Read the model definition and answer for the solid it produces. Units are mm, in the model's axes. A direction names the side the tool comes from. Round coordinates to 2 decimals unless told otherwise and drop trailing zeros. Write each loop counter-clockwise with the first axis right and the second up, starting at its lowest first coordinate (ties: lowest second). Pieces come first, ordered by that corner, then holes. Notation, with made-up numbers: (55.5, 18.25) -> (69.5, 18.25) arc R35 cw to (69.5, 54.25) -> close; hole circle Ø11 at (88.25, -37). An arc over 180 degrees is marked (long way). Return JSON: item names as keys, results as strings.
from build123d import *

# Parameters (mm, degrees)
SKETCH1_W             = 76
SKETCH1_H             = 62
BOSS_EXTRUDE1_DEPTH   = 2
SKETCH2_W             = 82
SKETCH2_H             = 68
BOSS_EXTRUDE2_DEPTH   = 8
SKETCH3_W             = 45
SKETCH3_H             = 12.8
CUT_EXTRUDE1_DEPTH    = 11
SKETCH4_R             = 1.6
CUT_EXTRUDE2_DEPTH    = 11
SKETCH5_R             = 3.1
CUT_EXTRUDE3_DEPTH    = 3
SKETCH9_OUTSIDE_W     = 105.4
SKETCH9_OUTSIDE_H     = 91.4
SKETCH9_OUTSIDE_W_2   = 75.6
SKETCH9_OUTSIDE_H_2   = 61.6
CUT_EXTRUDE5_DEPTH    = 3
CUT_EXTRUDE6_DEPTH    = 3
SKETCH11_W            = 66
SKETCH11_H            = 54
CUT_EXTRUDE7_DEPTH    = 7
CHAMFER2_SIZE         = 2
CHAMFER2_SIZE2        = 0.352653961
CHAMFER2_PART_2_SIZE  = 2
CHAMFER2_PART_2_SIZE2 = 0.352653961
CHAMFER3_SIZE         = 1
CHAMFER3_SIZE2        = 1.732050808


with BuildPart() as part:
    # Sketch1 → Boss-Extrude1 (new body)
    with BuildSketch(Plane(origin=(0, 0, 0), x_dir=(1, 0, 0), z_dir=(0, 1, 0))):
        Rectangle(SKETCH1_W, SKETCH1_H)
    extrude(amount=BOSS_EXTRUDE1_DEPTH)

    # Sketch2 → Boss-Extrude2 (add)
    with BuildSketch(Plane(origin=(0, 2, 0), x_dir=(1, 0, 0), z_dir=(0, 1, 0))):
        Rectangle(SKETCH2_W, SKETCH2_H)
    extrude(amount=BOSS_EXTRUDE2_DEPTH)

    # Sketch3 → Cut-Extrude1 (cut, through all)
    with BuildSketch(Plane.XZ):
        with Locations((0, -12.5)):
            Rectangle(SKETCH3_W, SKETCH3_H)
        with Locations((0, 12.5)):
            Rectangle(SKETCH3_W, SKETCH3_H)
    extrude(amount=-CUT_EXTRUDE1_DEPTH, mode=Mode.SUBTRACT)

    # Sketch4 → Cut-Extrude2 (cut, through all)
    with BuildSketch(Plane(origin=(0, 10, 0), x_dir=(1, 0, 0), z_dir=(0, 1, 0))):
        with Locations(Location((-35.408866178, 29.363450001, 0), (0, 0, 270))):  # turned: the seam where the file's is
            Circle(SKETCH4_R)
        with Locations(Location((35.408866178, 29.363450001, 0), (0, 0, 270))):  # turned: the seam where the file's is
            Circle(SKETCH4_R)
        with Locations(Location((35.408866178, -29.363450001, 0), (0, 0, 270))):  # turned: the seam where the file's is
            Circle(SKETCH4_R)
        with Locations(Location((-35.408866178, -29.363450001, 0), (0, 0, 270))):  # turned: the seam where the file's is
            Circle(SKETCH4_R)
    extrude(amount=-CUT_EXTRUDE2_DEPTH, mode=Mode.SUBTRACT)

    # Sketch5 → Cut-Extrude3 (cut)
    with BuildSketch(Plane(origin=(0, 10, 0), x_dir=(1, 0, 0), z_dir=(0, 1, 0))):
        with Locations(Location((-35.408866178, 29.363450001, 0), (0, 0, 270))):  # turned: the seam where the file's is
            Circle(SKETCH5_R)
        with Locations(Location((35.408866178, 29.363450001, 0), (0, 0, 270))):  # turned: the seam where the file's is
            Circle(SKETCH5_R)
        with Locations(Location((35.408866178, -29.363450001, 0), (0, 0, 270))):  # turned: the seam where the file's is
            Circle(SKETCH5_R)
        with Locations(Location((-35.408866178, -29.363450001, 0), (0, 0, 270))):  # turned: the seam where the file's is
            Circle(SKETCH5_R)
    extrude(amount=-CUT_EXTRUDE3_DEPTH, mode=Mode.SUBTRACT)

    # Sketch9 outside → Cut-Extrude5 (cut)
    with BuildSketch(Plane.XZ):
        Rectangle(SKETCH9_OUTSIDE_W, SKETCH9_OUTSIDE_H)
        Rectangle(SKETCH9_OUTSIDE_W_2, SKETCH9_OUTSIDE_H_2, mode=Mode.SUBTRACT)
    extrude(amount=-CUT_EXTRUDE5_DEPTH, mode=Mode.SUBTRACT)

    # Sketch10 → Cut-Extrude6 (cut)
    with BuildSketch(Plane.XZ):
        Polygon((-37.8, -30.8), (-31.8, -30.8), (-37.8, -24.8), align=None)
        Polygon((-37.8, 24.8), (-37.8, 30.8), (-31.8, 30.8), align=None)
        Polygon((37.8, 30.8), (37.8, 24.8), (31.8, 30.8), align=None)
        Polygon((37.8, -30.8), (31.8, -30.8), (37.8, -24.8), align=None)
    extrude(amount=-CUT_EXTRUDE6_DEPTH, mode=Mode.SUBTRACT)

    # Sketch11 → Cut-Extrude7 (cut)
    with BuildSketch(Plane.XZ):
        Rectangle(SKETCH11_W, SKETCH11_H)
    extrude(amount=-CUT_EXTRUDE7_DEPTH, mode=Mode.SUBTRACT)

    # Chamfer2
    chamfer2_edges = [part.edges().sort_by_distance(p)[0] for p in [
        (37.8, 0, 0),
    ]]
    chamfer2_side = [part.faces().sort_by_distance(p)[0] for p in [
        (37.8, 1.5, 0),
    ]]
    chamfer(chamfer2_edges, length=CHAMFER2_SIZE, length2=CHAMFER2_SIZE2, reference=chamfer2_side[0])

    # Chamfer2 part 2
    chamfer2_part_2_edges = [part.edges().sort_by_distance(p)[0] for p in [
        (-37.8, 0, 0),
    ]]
    chamfer2_part_2_side = [part.faces().sort_by_distance(p)[0] for p in [
        (-37.8, 1.5, 0),
    ]]
    chamfer(chamfer2_part_2_edges, length=CHAMFER2_PART_2_SIZE, length2=CHAMFER2_PART_2_SIZE2, reference=chamfer2_part_2_side[0])

    # Chamfer3
    chamfer3_edges = [part.edges().sort_by_distance(p)[0] for p in [
        (0, 0, -30.8),
        (0, 0, 30.8),
    ]]
    chamfer3_side = [part.faces().sort_by_distance(p)[0] for p in [
        (-35.357643735, 0, 25.870950059),
    ]]
    chamfer(chamfer3_edges, length=CHAMFER3_SIZE, length2=CHAMFER3_SIZE2, reference=chamfer3_side[0])


solid = part.part
Item 1: Section C-C (x = 28) is taken. Give the vertices of the cut face in (y, z).
Worked answers:
{"outline": "(0, -29.8) -> (1.73, -30.8) -> (3, -30.8) -> (3, -34) -> (10, -34) -> (10, 34) -> (3, 34) -> (3, 30.8) -> (1.73, 30.8) -> (0, 29.8) -> (0, 27) -> (7, 27) -> (7, -27) -> (0, -27) -> close"}
Item 2: Section A-A (z = 9) is taken. Give the vertices of the cut face in (x, y), then the cut area to 3 significant figures.
Worked answers:
{"outline": "(-41, 3) -> (-37.8, 3) -> (-37.8, 2) -> (-37.45, 0) -> (-33, 0) -> (-33, 7) -> (-22.5, 7) -> (-22.5, 10) -> (-41, 10) -> close; (22.5, 7) -> (33, 7) -> (33, 0) -> (37.45, 0) -> (37.8, 2) -> (37.8, 3) -> (41, 3) -> (41, 10) -> (22.5, 10) -> close", "area": "203 mm2"}
Item 3: Section D-D (y = 5.5) is taken. Give the vertices of the cut face in (x, z).
Worked answers:
{"outline": "(-41, -34) -> (41, -34) -> (41, 34) -> (-41, 34) -> close; hole circle Ø3.2 at (-35.41, -29.36); hole circle Ø3.2 at (-35.41, 29.36); hole (-33, -27) -> (33, -27) -> (33, 27) -> (-33, 27) -> close; hole circle Ø3.2 at (35.41, -29.36); hole circle Ø3.2 at (35.41, 29.36)"}
Item 4: Flat-ended cylindrical pins translate along their axes: pin 1 (4 mm diameter, centred on x = 35.41, z = 29.36, fed in from +Y); pin 2 (6 mm diameter, centred on x = 14, z = 11.5, fed in from +Y). Find the tip coordinate at first contact, or state that the pin passes through.
Worked answers:
{"pin 1": "stops at y = 7", "pin 2": "passes through"}
Item 5: Section B-B (x = 3) is taken. Give the vertices of the cut face in (y, z).
Worked answers:
{"outline": "(0, -29.8) -> (1.73, -30.8) -> (3, -30.8) -> (3, -34) -> (10, -34) -> (10, -18.9) -> (7, -18.9) -> (7, -27) -> (0, -27) -> close; (0, 27) -> (7, 27) -> (7, 18.9) -> (10, 18.9) -> (10, 34) -> (3, 34) -> (3, 30.8) -> (1.73, 30.8) -> (0, 29.8) -> close; (7, -6.1) -> (10, -6.1) -> (10, 6.1) -> (7, 6.1) -> close"}
Item 6: A tool of negligible diameter and unlimited length cuts with its end or side. For faces 4 (the flat face through (32.9, 1.5, -29.7)), 5 (the flat face through (22.5, 8, 12)), 6 (the flat face through (0, 3, 27)), 7 (the flat face through (-37, 7, -28)), from which of +Z, -Z, +X, -X, +Y, -Y can it reach the whole face along a straight path? Write none if from no direction.
Worked answers:
{"face 4": "-Z, +X, -Y", "face 5": "+Y, -Y", "face 6": "-Y", "face 7": "+Y"}
Item 7: Straight lines are drawn through the part: L1, parallel to Z at x = 5, y = 9.5; L2, parallel to Z at x = 10.5, y = 4.75; L3, parallel to X at y = 2.75, z = 20. For each, find the intervals that lie inside material, in ascending order. Write a range as [from, to].
Worked answers:
{"L1": "z = [-34, -18.9], [-6.1, 6.1], [18.9, 34]", "L2": "z = [-34, -27], [27, 34]", "L3": "x = [-37.8, -33], [33, 37.8]"}
Item 8: For a pull along Z with two mould halves and no side action, classify faces 1 (the flat face through (-32.9, 1.5, 29.7)), 2 (the flat face through (0, 8, 18.9)), 3 (the flat face through (-37.62, 0.99, -0.35)) as released by +Z, released by -Z, zero draft, split by the parting line, or undercut.
Worked answers:
{"face 1": "released by +Z", "face 2": "undercut", "face 3": "zero draft"}
